Autodesk Inventor part; units mm, degrees
ref_plane "Work Plane2" through (0, 0, 41.5) normal (0, 0, 1) x (1, 0, 0)
ref_plane "YZ Plane" through (0, 0, 0) normal (1, 0, 0) x (0, 1, 0)
ref_plane "XZ Plane" through (0, 0, 0) normal (0, 1, 0) x (-1, 0, 0)
sketch "Sketch1" plane through (0, 0, 0) normal (0, 0, 1) x (1, 0, 0)
  circle A0 centre (0, 0) radius 3
  dimension "d0" = 6
extrude "Extrusion1" add sketch "Sketch1" along normal mid plane 80
sketch "Sketch2" plane through (0, 0, 40) normal (0, 0, 1) x (1, 0, 0)
  circle A0 centre (0, 0) radius 5
  dimension "d3" = 10
extrude "Extrusion2" add sketch "Sketch2" along normal blind 6
thread "Thread1"
sketch "Sketch3" plane through (0, 0, 46) normal (0, 0, 1) x (1, 0, 0)
  circle A0 centre (0, 0) radius 3
  line L0 (1.4434, 2.5) -> (2.8868, 0)
  line L1 (2.8868, 0) -> (1.4434, -2.5)
  line L2 (1.4434, -2.5) -> (-1.4434, -2.5)
  line L3 (-1.4434, -2.5) -> (-2.8868, 0)
  line L4 (-2.8868, 0) -> (-1.4434, 2.5)
  line L5 (-1.4434, 2.5) -> (1.4434, 2.5)
  dimension "d8" = 5
extrude "Extrusion3" cut sketch "Sketch3" against normal blind 3 contours L0 L1 L2 L3 L4 L5
ref_plane "Work Plane2" through (0, 0, 41.5) normal (0, 0, 1) x (1, 0, 0)
sketch "Sketch5" plane through (0, 0, 41.5) normal (0, 0, 1) x (1, 0, 0)
  point P0 (0, 0)
  point P1 (0, 0)
sketch "Sketch6" plane through (0, 0, 43) normal (0, 0, 1) x (1, 0, 0)
  circle A0 centre (0, 0) radius 2.5
  dimension "d13" = 5
loft "Loft1" cut profiles "Sketch6" section 2 point at (0, 0, 41.5)
properties part number "HCMUTE-CDT23-M6X80_SUOT" material "Stainless Steel"
Geometry check sheet. Reference: the model listing, model coordinates, mm. A direction names the side the tool comes from. Coordinates: 2 decimals unless noted, no trailing zeros. Order: outer loops, then holes, each group sorted by start corner. A loop starts at its lowest first (then second) coordinate and runs counter-clockwise, first axis right, second up.
Q1. Sectioned sample at A-A on x = 4. Record the cut outline in (y, z).
Reply:
outline: (-3, 40) - (3, 40) - (3, 46) - (-3, 46) - close
Q2. Draft check along X on faces 4 (the face through (0, 0, -40)), 5 (the face through (-2.155, -1.267, 44.521)), 6 (the face through (-3, 0, 1)). Enter one of: released by +X, released by -X, zero draft, split by the parting line, or undercut.
Reply:
face 4: zero draft
face 5: undercut
face 6: split by the parting line
Q3. Tool access check on faces 1 (the face through (3.3, 0.1, 40)), 2 (the face through (-1.08, 4.88, 42.96)), 3 (the face through (0, -2.5, 45)). Record the directions out of +Z, -Z, +X, -X, +Y, -Y that give a thin tool (end or side, any length) a straight path to the whole face; none if there is none.
Reply:
face 1: -Z
face 2: +Z, -Z
face 3: +Z
Q4. Depth check by flat-ended pin: pin 1 Ø3 at (x, z) = (2, 6) entering from -Y; pin 2 Ø2 at (x, z) = (3, -1) entering from +Y; pin 3 Ø0.6 at (x, y) = (1, 1.5) entering from +Z. Enter the tip coordinate at first touch or a pass-through.
Reply:
pin 1: stops at y = -2.96
pin 2: stops at y = 2.24
pin 3: stops at z = 42.76
Q5. Thickness scan on probe 1 along Y at (x, z) = (0.75, -24); probe 2 along Z at (x, y) = (-2.5, 3); probe 3 along Z at (x, y) = (2.5, -0.5). Record the ranges inside material, lowest first.
Reply:
probe 1: y = -2.9 to 2.9
probe 2: z = 40 to 46
probe 3: z = -40 to 43
Q6. Sectioned sample at B-B on z = 2. Record the cut outline in (x, y).
Reply:
outline: circle Ø6 at (0, 0)
